Design review of the part built by this model. Coordinates are the model's own, in mm. A direction names the side the tool comes from. Coordinates: 2 decimals unless noted, no trailing zeros. Write each loop counter-clockwise with the first axis right and the second up, starting at its lowest first coordinate (ties: lowest second). Pieces come first, ordered by that corner, then holes.
Q1. For faces 5 (the flat face through (17, 31, -5)), 6 (the flat face through (5, 0, 0)), 7 (the flat face through (3, -18.14, 0)), list the 3-axis set-ups (+Z, -Z, +X, -X, +Y, -Y) from which the entire face can be reached by the end or side of a thin tool; tool diameter is ignored.
Q2. Take a section at D-D, the plane y = -13.14. Write out the cut boundary in (x, z).
Q3. Take a section at B-B, the plane y = 0. Write out the cut boundary in (x, z), plus the area to 3 significant figures.
Q4. For L1, parallel to Y at x = 3.8, z = 0; L2, parallel to Y at x = 3, z = 14; L3, parallel to Y at x = 2.75, z = -13.14, list the stretches that pass through material, from the lowest coordinate up.
Q5. For pin 1 Ø3 at (y, z) = (26.5, 27.5) entering from +X; pin 2 Ø2 at (x, z) = (1.5, -12.5) entering from +Y; pin 3 Ø2.5 at (y, z) = (34.59, 0) entering from -X; pin 4 Ø1.5 at (x, y) = (3.5, -8.5) entering from +Z, all flat-tipped, find the tip position at first contact; note any pin that passes through.
Q6. The part is to be moulded in two halves that separate along Y. For faces 1 (the flat face through (3, -8.14, 0)), 2 (the flat face through (0, 1, 1)), 3 (the cylindrical face through (8.38, 37.18, 4.88)), 4 (the cylindrical face through (2.46, 13.98, -12.6)), say which applies: released by +Y, released by -Y, zero draft, split by the parting line, or undercut.
Q7. Take a section at A-A, the plane z = 0. Write out the cut boundary in (x, y).
Q8. Take a section at C-C, the plane z = -13.14. Write out the cut boundary in (x, y), plus the area to 3 significant figures.
from build123d import *

# Parameters (mm, degrees)
SKETCH1_R               = 37.5
BOSS_EXTRUDE1_DEPTH     = 5
SKETCH3_R               = 1
CUT_EXTRUDE2_DEPTH      = 6
SKETCH4_R               = 37.5
SKETCH4_R_2             = 31
BOSS_EXTRUDE2_DEPTH     = 12
SKETCH2_R               = 1.3
CUT_EXTRUDE1_DEPTH      = 13
CUT_EXTRUDE1_DEPTH_BACK = 6
CUT_EXTRUDE3_DEPTH      = 6


with BuildPart() as part:
    # Sketch1 → Boss-Extrude1 (new body)
    with BuildSketch(Plane(origin=(0, 0, 0), x_dir=(0, 0, -1), z_dir=(1, 0, 0))):
        Circle(SKETCH1_R)
    extrude(amount=BOSS_EXTRUDE1_DEPTH)

    # Sketch3 → Cut-Extrude2 (cut, through all)
    with BuildSketch(Plane.ZY):
        with Locations((-13.14, 13.14)):
            Circle(SKETCH3_R)
        with Locations((13.14, 13.14)):
            Circle(SKETCH3_R)
        with Locations((13.14, -13.14)):
            Circle(SKETCH3_R)
        with Locations((-13.14, -13.14)):
            Circle(SKETCH3_R)
    extrude(amount=-CUT_EXTRUDE2_DEPTH, mode=Mode.SUBTRACT)

    # Sketch4 → Boss-Extrude2 (add)
    with BuildSketch(Plane(origin=(5, 0, 0), x_dir=(0, 0, -1), z_dir=(1, 0, 0))):
        Circle(SKETCH4_R)
        Circle(SKETCH4_R_2, mode=Mode.SUBTRACT)
    extrude(amount=BOSS_EXTRUDE2_DEPTH)

    # Sketch2 → Cut-Extrude1 (cut, two sides)
    with BuildSketch(Plane(origin=(5, 0, 0), x_dir=(0, 0, -1), z_dir=(1, 0, 0))) as cut_extrude1_sk:
        with Locations((0, 34.588098227)):
            Circle(SKETCH2_R)
        with Locations((8.984441127, -33.400843651)):
            Circle(SKETCH2_R)
        with Locations((34.588098227, 0)):
            Circle(SKETCH2_R)
        with Locations((-33.400843651, -8.984441127)):
            Circle(SKETCH2_R)
    extrude(amount=CUT_EXTRUDE1_DEPTH, mode=Mode.SUBTRACT)
    extrude(cut_extrude1_sk.sketch, amount=-CUT_EXTRUDE1_DEPTH_BACK, mode=Mode.SUBTRACT)

    # Sketch5 → Cut-Extrude3 (cut, through all)
    with BuildSketch(Plane(origin=(5, 0, 0), x_dir=(0, 0, -1), z_dir=(1, 0, 0))):
        with BuildLine():
            Line((9.75, -8.14), (-9.75, -8.14))
            ThreePointArc((-9.75, -8.14), (-10.457106781, -8.432893219), (-10.75, -9.14))
            Line((-10.75, -9.14), (-10.75, -17.14))
            ThreePointArc((-10.75, -17.14), (-10.457106781, -17.847106781), (-9.75, -18.14))
            Line((-9.75, -18.14), (9.75, -18.14))
            ThreePointArc((9.75, -18.14), (10.457106781, -17.847106781), (10.75, -17.14))
            Line((10.75, -17.14), (10.75, -12.14))
            ThreePointArc((10.75, -12.14), (11.042893219, -11.432893219), (11.75, -11.14))
            Line((11.75, -11.14), (14.53, -11.14))
            ThreePointArc((14.53, -11.14), (15.237106781, -10.847106781), (15.53, -10.14))
            Line((15.53, -10.14), (15.53, -4.14))
            ThreePointArc((15.53, -4.14), (15.237106781, -3.432893219), (14.53, -3.14))
            Line((14.53, -3.14), (11.75, -3.14))
            ThreePointArc((11.75, -3.14), (11.042893219, -3.432893219), (10.75, -4.14))
            Line((10.75, -4.14), (10.75, -7.14))
            ThreePointArc((10.75, -7.14), (10.457106781, -7.847106781), (9.75, -8.14))
        make_face()
    extrude(amount=-CUT_EXTRUDE3_DEPTH, mode=Mode.SUBTRACT)


solid = part.part
Responses:
1. face 5: +Z, -Z, +X, +Y, -Y
1. face 6: +X
1. face 7: +X, -X
2. outline: (0, -35.12) - (17, -35.12) - (17, -28.08) - (5, -28.08) - (5, -14.14) - (0, -14.14) - close; (0, -12.14) - (5, -12.14) - (5, -10.75) - (0, -10.75) - close; (0, 10.75) - (5, 10.75) - (5, 12.14) - (0, 12.14) - close; (0, 14.14) - (5, 14.14) - (5, 28.08) - (17, 28.08) - (17, 35.12) - (0, 35.12) - close
3. outline: (0, -37.5) - (17, -37.5) - (17, -35.89) - (0, -35.89) - close; (0, -33.29) - (17, -33.29) - (17, -31) - (5, -31) - (5, 31) - (17, 31) - (17, 37.5) - (0, 37.5) - close
3. area: 487 mm2
4. L1: y = -37.5 to -18.14, -8.14 to 33.29, 35.89 to 37.5
4. L2: y = -34.79 to -13.65, -12.63 to 12.63, 13.65 to 34.79
4. L3: y = -35.12 to -14.14, -12.14 to -11.14, -3.14 to 12.14, 14.14 to 35.12
5. pin 1: stops at x = 17
5. pin 2: stops at y = 35.69
5. pin 3: passes through
5. pin 4: stops at z = 36.69
6. face 1: undercut
6. face 2: zero draft
6. face 3: split by the parting line
6. face 4: undercut
7. outline: (0, -37.5) - (17, -37.5) - (17, -31) - (5, -31) - (5, -18.14) - (0, -18.14) - close; (0, -8.14) - (5, -8.14) - (5, 31) - (17, 31) - (17, 33.29) - (0, 33.29) - close; (0, 35.89) - (17, 35.89) - (17, 37.5) - (0, 37.5) - close
8. outline: (0, -35.12) - (17, -35.12) - (17, -28.08) - (5, -28.08) - (5, -14.14) - (0, -14.14) - close; (0, -12.14) - (5, -12.14) - (5, -11.14) - (0, -11.14) - close; (0, -3.14) - (5, -3.14) - (5, 12.14) - (0, 12.14) - close; (0, 14.14) - (5, 14.14) - (5, 28.08) - (17, 28.08) - (17, 35.12) - (0, 35.12) - close
8. area: 460 mm2
